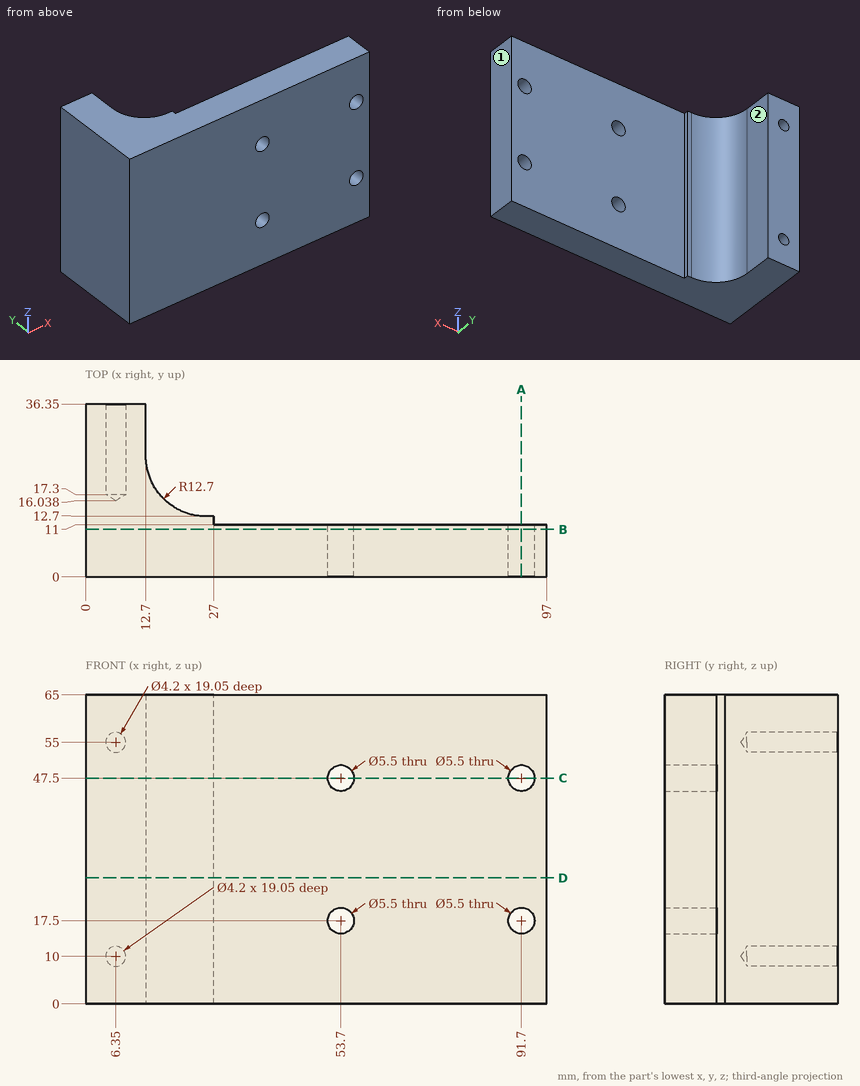
Geometry check sheet. Reference: drawing and pictorial views, mm from the part's lowest x, y, z. A direction names the side the tool comes from. Round coordinates to 2 decimals unless told otherwise and drop trailing zeros. Write each loop counter-clockwise with the first axis right and the second up, starting at its lowest first coordinate (ties: lowest second). Pieces come first, ordered by that corner, then holes.
1. Section check D-D on z = 26.5. Enter the section's corners in (x, y).
2. Section check B-B on y = 10. Enter the section's corners in (x, z), plus the area to 3 significant figures.
3. Access from +Z, -Z, +X, -X, +Y, -Y to the whole of each face (thin tool, end or side, straight path). Record for the marked faces 1 and 2.
4. Section check C-C on z = 47.5. Enter the section's corners in (x, y), plus the area to 3 significant figures.
5. Scan lines: L1, parallel to Z at x = 6.35, y = 23; L2, parallel to Z at x = 53.7, y = 3.75; L3, parallel to X at y = 8, z = 17. Record each from-to range of solid material in increasing order.
6. Section check A-A on x = 91.7. Enter the section's corners in (y, z).
7. Gauge pin test, flat ends, axial feed: P1, Ø1.9, axis at y = 12, z = 20, coming from the +X side; P2, Ø1.8, axis at x = 26.5, z = 29.5, coming from the +Y side; P3, Ø19.5, axis at x = 67, z = 43, coming from the +Y side. Record the tip position at first contact, or that the pin passes through.
Answer:
1. outline: (0, 0) - (97, 0) - (97, 11) - (27, 11) - (27, 12.7) - (25.4, 12.7) arc R12.7 cw to (12.7, 25.4) - (12.7, 36.35) - (0, 36.35) - close
2. outline: (0, 0) - (97, 0) - (97, 65) - (0, 65) - close; hole circle Ø5.5 at (53.7, 17.5); hole circle Ø5.5 at (53.7, 47.5); hole circle Ø5.5 at (91.7, 17.5); hole circle Ø5.5 at (91.7, 47.5)
2. area: 6,210 mm2
3. face 1: +Z, -Z, +X, +Y, -Y
3. face 2: +Z, -Z, +X, +Y
4. outline: (0, 0) - (50.95, 0) - (50.95, 11) - (27, 11) - (27, 12.7) - (25.4, 12.7) arc R12.7 cw to (12.7, 25.4) - (12.7, 36.35) - (0, 36.35) - close; (56.45, 0) - (88.95, 0) - (88.95, 11) - (56.45, 11) - close; (94.45, 0) - (97, 0) - (97, 11) - (94.45, 11) - close
4. area: 1,330 mm2
5. L1: z = 0 to 7.9, 12.1 to 52.9, 57.1 to 65
5. L2: z = 0 to 14.75, 20.25 to 44.75, 50.25 to 65
5. L3: x = 0 to 51, 56.4 to 89, 94.4 to 97
6. outline: (0, 0) - (11, 0) - (11, 14.75) - (0, 14.75) - close; (0, 20.25) - (11, 20.25) - (11, 44.75) - (0, 44.75) - close; (0, 50.25) - (11, 50.25) - (11, 65) - (0, 65) - close
7. P1: stops at x = 27
7. P2: stops at y = 12.7
7. P3: stops at y = 11
